Can you work these out from the model? Positions are in its coordinate system, mm. A direction names the side the tool comes from. Give positions to 0.01 mm unless a question says otherwise; leave off trailing zeros. Order: outer loops, then holes, each group sorted by start corner. A loop starts at its lowest first (then second) coordinate and runs counter-clockwise, first axis right, second up. Notation, with made-up numbers: (42, 8.25) - (47, 8.25) arc R27 ccw to (47, 30.25) - close; hole circle Ø1 at (-18, -4). An arc over 180 degrees is marked (long way). One line per question, with ' | ' between items.
```python
from build123d import *

# Parameters (mm, degrees)
SKETCH4_W                    = 136.525
SKETCH4_H                    = 15.875
SKETCH4_W_2                  = 44.45
SKETCH4_H_2                  = 14.2875
BOSS_EXTRUDE2_DEPTH          = 6.35
FILLET4_R                    = 4.7625
FILLET5_R                    = 6.35
CUT_EXTRUDE3_DEPTH           = 6.35
F_18_0_1695_DIAMETER_HOLE1_D = 4.3053
F_18_0_1695_DIAMETER_HOLE2_D = 4.3053
LPATTERN1_COUNT              = 2
LPATTERN1_PITCH              = 41.275
F_0_257_DIAMETER_HOLE1_D     = 6.5278
SKETCH5_R                    = 11
CUT_EXTRUDE4_DEPTH           = 7.35
LPATTERN2_COUNT              = 2
LPATTERN2_PITCH              = 98.425
MIRROR1_COPY_1_DEPTH         = 6.35
MIRROR1_COPY_2_DEPTH         = 6.35
SKETCH20_R                   = 1.8288
CUT_EXTRUDE5_DEPTH           = 7.35


with BuildPart() as part:
    # Sketch4 → Boss-Extrude2 (new body)
    with BuildSketch(Plane.XY):
        Polygon((-158.75, -22.225), (-158.75, -7.9375), (-158.75, 7.9375), (-158.75, 22.225), (-171.45, 22.225), (-171.45, -22.225), align=None)
        with Locations((-90.4875, 0)):
            Rectangle(SKETCH4_W, SKETCH4_H)
        with Locations((0, 15.08125)):
            Rectangle(SKETCH4_W_2, SKETCH4_H_2)
        Rectangle(SKETCH4_W_2, SKETCH4_H)
        with Locations((0, -15.08125)):
            Rectangle(SKETCH4_W_2, SKETCH4_H_2)
        with Locations((90.4875, 0)):
            Rectangle(SKETCH4_W, SKETCH4_H)
        Polygon((158.75, 7.9375), (158.75, -7.9375), (158.75, -22.225), (171.45, -22.225), (171.45, 22.225), (158.75, 22.225), align=None)
    extrude(amount=BOSS_EXTRUDE2_DEPTH)

    # Fillet4
    fillet4_edges = [part.edges().sort_by_distance(p)[0] for p in [
        (-158.75, 7.9375, 3.175),
        (-22.225, 7.9375, 3.175),
        (22.225, 7.9375, 3.175),
        (158.75, 7.9375, 3.175),
        (158.75, -7.9375, 3.175),
        (22.225, -7.9375, 3.175),
        (-22.225, -7.9375, 3.175),
        (-158.75, -7.9375, 3.175),
    ]]
    fillet(fillet4_edges, radius=FILLET4_R)

    # Fillet5
    fillet5_edges = [part.edges().sort_by_distance(p)[0] for p in [
        (-158.75, 22.225, 3.175),
        (-22.225, 22.225, 3.175),
        (22.225, 22.225, 3.175),
        (158.75, 22.225, 3.175),
        (158.75, -22.225, 3.175),
        (22.225, -22.225, 3.175),
        (-22.225, -22.225, 3.175),
        (-158.75, -22.225, 3.175),
    ]]
    fillet(fillet5_edges, radius=FILLET5_R)

    # Sketch7 → Cut-Extrude3 (cut)
    with BuildSketch(Plane.XY.offset(6.35)):
        with BuildLine():
            Line((-153.194004, 2.38125), (-126.205996004, 2.38125))
            ThreePointArc((-126.205996004, 2.38125), (-124.522377586, 1.683872418), (-123.825000004, 0.000254))
            ThreePointArc((-123.825000004, 0.000254), (-124.522377586, -1.683872418), (-126.205996004, -2.38125))
            Line((-126.205996004, -2.38125), (-153.194004, -2.38125))
            ThreePointArc((-153.194004, -2.38125), (-154.877622418, -1.683872418), (-155.575, 0.000254))
            ThreePointArc((-155.575, 0.000254), (-154.877622418, 1.683872418), (-153.194004, 2.38125))
        make_face()
    cut_extrude3 = extrude(amount=-CUT_EXTRUDE3_DEPTH, mode=Mode.SUBTRACT)

    # #18 (0.1695) Diameter Hole1 (through all)
    with Locations(Plane.XY.offset(6.35)):
        with Locations((-165.1, 15.875), (-165.1, 0), (-165.1, -15.875)):
            f_18_0_1695_diameter_hole1 = Hole(F_18_0_1695_DIAMETER_HOLE1_D / 2)

    # #18 (0.1695) Diameter Hole2 (through all)
    with Locations(Plane(origin=(0, 0, 0), x_dir=(-1, 0, 0), z_dir=(0, 0, -1))):
        with Locations((-15.715448212, -15.715448212), (-15.715448212, 15.715448212)):
            f_18_0_1695_diameter_hole2 = Hole(F_18_0_1695_DIAMETER_HOLE2_D / 2)

    # LPattern1: Cut-Extrude3 ×2
    with Locations(*[(i * LPATTERN1_PITCH, 0, 0) for i in range(1, LPATTERN1_COUNT)]):
        add(cut_extrude3, mode=Mode.SUBTRACT)

    # F (0.257) Diameter Hole1 (through all)
    with Locations(Plane(origin=(0, 0, 0), x_dir=(-1, 0, 0), z_dir=(0, 0, -1))):
        with Locations((-69.85, 0)):
            f_0_257_diameter_hole1 = Hole(F_0_257_DIAMETER_HOLE1_D / 2)

    # Sketch5 → Cut-Extrude4 (cut, through all)
    with BuildSketch(Plane.XY.offset(6.35)):
        Circle(SKETCH5_R)
    extrude(amount=-CUT_EXTRUDE4_DEPTH, mode=Mode.SUBTRACT)

    # LPattern2: Cut-Extrude3 ×2
    with Locations(*[(i * LPATTERN2_PITCH, 0, 0) for i in range(1, LPATTERN2_COUNT)]):
        add(cut_extrude3, mode=Mode.SUBTRACT)

    # Mirror1: #18 (0.1695) Diameter Hole2, #18 (0.1695) Diameter Hole1, F (0.257) Diameter Hole1, Cut-Extrude3 across plane
    add(f_18_0_1695_diameter_hole2.mirror(Plane(origin=(0, 0, 0), x_dir=(0, 0, 1), z_dir=(1, 0, 0))), mode=Mode.SUBTRACT)
    add(f_18_0_1695_diameter_hole1.mirror(Plane(origin=(0, 0, 0), x_dir=(0, 0, 1), z_dir=(1, 0, 0))), mode=Mode.SUBTRACT)
    add(f_0_257_diameter_hole1.mirror(Plane(origin=(0, 0, 0), x_dir=(0, 0, 1), z_dir=(1, 0, 0))), mode=Mode.SUBTRACT)
    add(cut_extrude3.mirror(Plane(origin=(0, 0, 0), x_dir=(0, 0, 1), z_dir=(1, 0, 0))), mode=Mode.SUBTRACT)

    # Mirror1 copy 1 sketch → Mirror1 copy 1 (cut)
    with BuildSketch(Plane(origin=(-98.425, 0, 6.35), x_dir=(-1, 0, 0), z_dir=(0, 0, 1))):
        with BuildLine():
            Line((-153.194004, -2.38125), (-126.205996004, -2.38125))
            ThreePointArc((-126.205996004, -2.38125), (-124.522377586, -1.683872418), (-123.825000004, -0.000254))
            ThreePointArc((-123.825000004, -0.000254), (-124.522377586, 1.683872418), (-126.205996004, 2.38125))
            Line((-126.205996004, 2.38125), (-153.194004, 2.38125))
            ThreePointArc((-153.194004, 2.38125), (-154.877622418, 1.683872418), (-155.575, -0.000254))
            ThreePointArc((-155.575, -0.000254), (-154.877622418, -1.683872418), (-153.194004, -2.38125))
        make_face()
    extrude(amount=-MIRROR1_COPY_1_DEPTH, mode=Mode.SUBTRACT)

    # Mirror1 copy 2 sketch → Mirror1 copy 2 (cut)
    with BuildSketch(Plane(origin=(-41.275, 0, 6.35), x_dir=(-1, 0, 0), z_dir=(0, 0, 1))):
        with BuildLine():
            Line((-153.194004, -2.38125), (-126.205996004, -2.38125))
            ThreePointArc((-126.205996004, -2.38125), (-124.522377586, -1.683872418), (-123.825000004, -0.000254))
            ThreePointArc((-123.825000004, -0.000254), (-124.522377586, 1.683872418), (-126.205996004, 2.38125))
            Line((-126.205996004, 2.38125), (-153.194004, 2.38125))
            ThreePointArc((-153.194004, 2.38125), (-154.877622418, 1.683872418), (-155.575, -0.000254))
            ThreePointArc((-155.575, -0.000254), (-154.877622418, -1.683872418), (-153.194004, -2.38125))
        make_face()
    extrude(amount=-MIRROR1_COPY_2_DEPTH, mode=Mode.SUBTRACT)

    # Sketch20 → Cut-Extrude5 (cut, through all)
    with BuildSketch(Plane(origin=(0, 0, 0), x_dir=(-1, 0, 0), z_dir=(0, 0, -1))):
        with Locations((-119.062500002, -0.000254)):
            Circle(SKETCH20_R)
    cut_extrude5 = extrude(amount=-CUT_EXTRUDE5_DEPTH, mode=Mode.SUBTRACT)

    # Mirror2: Cut-Extrude5 across plane
    add(cut_extrude5.mirror(Plane(origin=(0, 0, 0), x_dir=(0, 0, 1), z_dir=(1, 0, 0))), mode=Mode.SUBTRACT)


solid = part.part
```
(1) On a 3-axis mill with a long thin cutter (end or side, diameter ignored), from which of +Z, -Z, +X, -X, +Y, -Y can I reach the whole of each face in a straight line? I mean faces 3 (the face through (160.561, -20.315, 3.219)), 4 (the face through (-41, 2.381, 3)), 5 (the face through (90, 7.938, 3)). Say none if no direction works.
Answer below:
face 3: +Z, -Z, -Y | face 4: +Z, -Z | face 5: +Z, -Z, +Y
(2) If I drill on line 1 (X direction, y = 12, z = 3.5); line 2 (X direction, y = 13.5, z = 5) (3 decimals); line 3 (Y direction, x = 37, z = 3.75), over which ranges is the centre line in solid material (lowest first)?
Answer below:
line 1: -171.45 to -158.7, -22.28 to 22.28, 158.7 to 171.45 | line 2: -171.45 to -158.75, -22.225 to 22.225, 158.75 to 171.45 | line 3: -7.94 to -2.38, 2.38 to 7.94
(3) Imagine slicing it at B-B (x = 0). List the corners of the cut face in (y, z) for me (3 decimals), and give its area (3 significant figures).
Answer below:
outline: (-22.225, 0) - (-11, 0) - (-11, 6.35) - (-22.225, 6.35) - close; (11, 0) - (22.225, 0) - (22.225, 6.35) - (11, 6.35) - close | area: 143 mm^2
(4) Imagine slicing it at A-A (x = 69.85). List the corners of the cut face in (y, z) for me, and give its area (3 significant figures).
Answer below:
outline: (-7.94, 0) - (-3.26, 0) - (-3.26, 6.35) - (-7.94, 6.35) - close; (3.26, 0) - (7.94, 0) - (7.94, 6.35) - (3.26, 6.35) - close | area: 59.4 mm^2
(5) If we mould it in two halves opening along X, with no side actions, what happens to faces 1 (the face through (-14, -2, 0)), 2 (the face through (-2.38, -10.74, 3.22))? For each: released by +X, released by -X, zero draft, split by the parting line, or undercut.
Answer below:
face 1: zero draft | face 2: undercut
(6) Imagine slicing it at C-C (z = 5.25). Count the separate pieces of the cut face and the enclosed holes in it, and give its area (3 significant figures).
Answer below:
separate pieces: 1 | enclosed holes: 21 | area: 5,920 mm^2
(7) Will these pins go through, and if not, where does the flat tip stop? pin 1 (2.5 mm diameter, centred on x = -15.72, y = 15.72, fed in from +Z); pin 2 (3 mm diameter, centred on x = 66.5, z = 2, fed in from +Y); pin 3 (1.9 mm diameter, centred on x = -44.5, z = 3.5, fed in from -Y).
Answer below:
pin 1: through | pin 2: y = 7.94 | pin 3: y = -7.94
